Build history of the part. All positions in model axes, mm. Round coordinates to 2 decimals unless told otherwise and drop trailing zeros. Loops run counter-clockwise (first coordinate to the right, second up) from the corner with the lowest first, then second, coordinate; pieces in that order, holes last. Notation, with made-up numbers: (47.5, 6) - (72.5, 6) arc R10 ccw to (72.5, 11) - close; hole circle Ø7 at (58.25, 56). An arc over 180 degrees is marked (long way). Answer as CSV lines item,"result". Start each with the question number.
```python
from build123d import *

# Parameters (mm, degrees)
SKETCH1_R               = 1.55
BOSS_EXTRUDE1_DEPTH     = 3
CUT_EXTRUDE2_DEPTH      = 71.677082566
CUT_EXTRUDE2_DEPTH_BACK = 71.677082566
SKETCH2_R               = 0.6


with BuildPart() as part:
    # Sketch1 → Boss-Extrude1 (new body)
    with BuildSketch(Plane(origin=(0, 0, 0), x_dir=(1, 0, 0), z_dir=(0, 1, 0))):
        with BuildLine():
            Line((-66.5, 4), (66.5, 4))
            ThreePointArc((66.5, 4), (70.5, 0), (66.5, -4))
            Line((66.5, -4), (-66.5, -4))
            ThreePointArc((-66.5, -4), (-70.5, 0), (-66.5, 4))
        make_face()
        with Locations(Location((-66.5, 0, 0), (0, 0, 270))):
            Circle(SKETCH1_R, mode=Mode.SUBTRACT)
        with Locations(Location((66.5, 0, 0), (0, 0, 90))):
            Circle(SKETCH1_R, mode=Mode.SUBTRACT)
    extrude(amount=BOSS_EXTRUDE1_DEPTH)

    # Sketch2 → Cut-Extrude2 (cut, two sides: drawn at the far end of the back side and taken through both)
    with BuildSketch(Plane(origin=(0, 0, 0), x_dir=(1, 0, 0), z_dir=(0, 1, 0)).offset(-CUT_EXTRUDE2_DEPTH_BACK)):
        with Locations(Location((0, 0, 0), (0, 0, 270))):
            Circle(SKETCH2_R)
    extrude(amount=CUT_EXTRUDE2_DEPTH + CUT_EXTRUDE2_DEPTH_BACK, mode=Mode.SUBTRACT)


solid = part.part
```
Q1. Wall check: probe 1 along X at (y, z) = (2.85, 0); probe 2 along Z at (x, y) = (66.5, 1.4); probe 3 along Z at (x, y) = (0, 1.9). Give the ranges that are in metal, low to high. Write a range as [from, to].
Q2. Two-plate mould, pull along Z, no slides. Class faces 1 (the flat face through (1, 3, 0)), 2 (the flat face through (-1, 1, -4)), 3 (the cylindrical face through (-64.963, 1.479, -0.202)): released by +Z, released by -Z, zero draft, split by the parting line, or undercut.
Q3. Pin check, flat tips, straight feed: pin 1 Ø2.5 at (x, z) = (66.5, 0) entering from -Y; pin 2 Ø1 at (y, z) = (1, -2.5) entering from +X. Stop position of each tip, or through.
Q4. Band-saw the part on B-B, the plane z = -2.75. List the corners of the cut face in (x, y).
Q5. Band-saw the part on A-A, the plane y = 1. List the corners of the cut face in (x, z), then the cut area to 3 significant figures.
Reported:
1,probe 1,"x = [-70.5, -68.05], [-64.95, -0.6], [0.6, 64.95], [68.05, 70.5]"
1,probe 2,"z = [-4, -1.55], [1.55, 4]"
1,probe 3,"z = [-4, -0.6], [0.6, 4]"
2,face 1,"zero draft"
2,face 2,"released by -Z"
2,face 3,"undercut"
3,pin 1,"passes through"
3,pin 2,"stops at x = 69.96"
4,outline,"(-69.4, 0) - (69.4, 0) - (69.4, 3) - (-69.4, 3) - close"
5,outline,"(-66.5, -4) - (66.5, -4) arc R4 ccw to (66.5, 4) - (-66.5, 4) arc R4 ccw to start; hole circle Ø3.1 at (-66.5, 0); hole circle Ø1.2 at (0, 0); hole circle Ø3.1 at (66.5, 0)"
5,area,"1,100 mm2"
